Model file for the job. Use its own axes, mm. Coordinates: 2 decimals unless noted, no trailing zeros. Order: outer loops, then holes, each group sorted by start corner. A loop starts at its lowest first (then second) coordinate and runs counter-clockwise, first axis right, second up. Notation, with made-up numbers: M 29.5,65.5 L 67.5,65.5 A22 ccw 67.5,83.5 Z; hole C 37,14 d2. An arc over 180 degrees is marked long. Return JSON: item names as keys, results as strings.
```python
from build123d import *

# Parameters (mm, degrees)
SKETCH1_W           = 246.38
SKETCH1_H           = 254
BOSS_EXTRUDE1_DEPTH = 2.54
SKETCH3_R           = 11.43
CUT_EXTRUDE1_DEPTH  = 3.54
LPATTERN1_COUNT     = 4
LPATTERN1_PITCH     = 60.96
SKETCH4_W           = 57.912
SKETCH4_H           = 254
CUT_EXTRUDE2_DEPTH  = 3.54


with BuildPart() as part:
    # Sketch1 → Boss-Extrude1 (new body)
    with BuildSketch(Plane.XY):
        Rectangle(SKETCH1_W, SKETCH1_H)
    extrude(amount=BOSS_EXTRUDE1_DEPTH)

    # Sketch3 → Cut-Extrude1 (cut, through all)
    with BuildSketch(Plane.XY.offset(2.54)):
        with Locations((-85.09, 109.22)):
            Circle(SKETCH3_R)
    cut_extrude1 = extrude(amount=-CUT_EXTRUDE1_DEPTH, mode=Mode.SUBTRACT)

    # LPattern1: Cut-Extrude1 ×4
    with Locations(*[(0, -i * LPATTERN1_PITCH, 0) for i in range(1, LPATTERN1_COUNT)]):
        add(cut_extrude1, mode=Mode.SUBTRACT)

    # Sketch4 → Cut-Extrude2 (cut, through all)
    with BuildSketch(Plane.XY.offset(2.54)):
        with Locations((94.234, 0)):
            Rectangle(SKETCH4_W, SKETCH4_H)
    extrude(amount=-CUT_EXTRUDE2_DEPTH, mode=Mode.SUBTRACT)


solid = part.part
```
Item 1: Saw through at C-C (z = 1.35). Write the cut outline in (x, y).
Check result:
{"outline": "M -123.19,-127 L 65.28,-127 L 65.28,127 L -123.19,127 Z; hole C -85.09,-73.66 d22.86; hole C -85.09,-12.7 d22.86; hole C -85.09,48.26 d22.86; hole C -85.09,109.22 d22.86"}
Item 2: Wall check: line 1 (Y direction, x = -85.09, z = 1.05); line 2 (X direction, y = -73, z = 1.95); line 3 (X direction, y = 43, z = 1.95). Give the ranges that are in metal, low to high.
Check result:
{"line 1": "y = -127 to -85.09, -62.23 to -24.13, -1.27 to 36.83, 59.69 to 97.79, 120.65 to 127", "line 2": "x = -123.19 to -96.5, -73.68 to 65.28", "line 3": "x = -123.19 to -95.24, -74.94 to 65.28"}
Item 3: Saw through at A-A (x = -85.09). Write the cut outline in (y, z).
Check result:
{"outline": "M -127,0 L -85.09,0 L -85.09,2.54 L -127,2.54 Z; M -62.23,0 L -24.13,0 L -24.13,2.54 L -62.23,2.54 Z; M -1.27,0 L 36.83,0 L 36.83,2.54 L -1.27,2.54 Z; M 59.69,0 L 97.79,0 L 97.79,2.54 L 59.69,2.54 Z; M 120.65,0 L 127,0 L 127,2.54 L 120.65,2.54 Z"}
Item 4: Pull direction Y, two halves, no side cores. Call faces 1 (the flat face through (-30, 2, 2.54)), 2 (the cylindrical face through (-79.816, -83.8, 1.288)), 3 (the cylindrical face through (-79.816, 99.08, 1.288)): +Y half, -Y half, draft (parallel to the pull), parting line (faces both ways), or undercut.
Check result:
{"face 1": "draft", "face 2": "undercut", "face 3": "undercut"}
Item 5: Saw through at B-B (y = -73.66). Write the cut outline in (x, z), and give its area (3 significant figures).
Check result:
{"outline": "M -123.19,0 L -96.52,0 L -96.52,2.54 L -123.19,2.54 Z; M -73.66,0 L 65.28,0 L 65.28,2.54 L -73.66,2.54 Z", "area": "421 mm2"}
Item 6: Saw through at D-D (y = -18.5). Write the cut outline in (x, z).
Check result:
{"outline": "M -123.19,0 L -94.94,0 L -94.94,2.54 L -123.19,2.54 Z; M -75.24,0 L 65.28,0 L 65.28,2.54 L -75.24,2.54 Z"}
